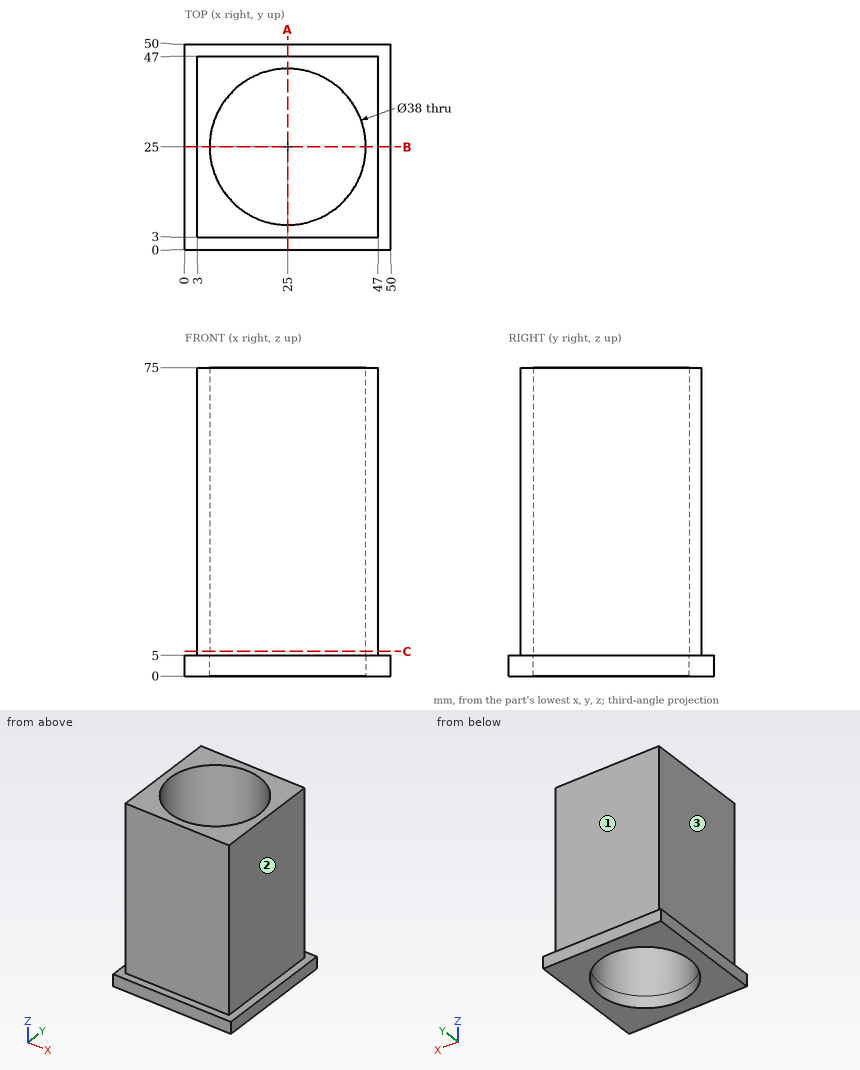
For this review, use the dimensioned drawing (mm, ordinates from the lowest corner) and the shaded views. A direction names the side the tool comes from. Coordinates: 2 decimals unless noted, no trailing zeros. Order: outer loops, then holes, each group sorted by start corner. A loop starts at its lowest first (then second) coordinate and runs counter-clockwise, first axis right, second up. Notation, with made-up numbers: M -19.5,-10 L 26.5,-10 A18 cw 26.5,6 Z; hole C 83.25,-22 d7. An arc over 180 degrees is marked long. Answer as a JSON object with one key per item and string values. Group by question number.
1) For pin 1 (6 mm diameter, centred on x = 24.5, z = 28.5, fed in from +Y); pin 2 (12 mm diameter, centred on x = 24.5, z = 29, fed in from -Y); pin 3 (12 mm diameter, centred on y = 15, z = 64.5, fed in from +X), all flat-tipped, find the tip position at first contact; note any pin that passes through.
2) Wall thickness on L1, parallel to Y at x = 25, z = 1; L2, parallel to Y at x = 25, z = 22.5; L3, parallel to Y at x = 45.5, z = 9: over which ranges is each line inside the solid? List them lowest first.
3) Tool access review of the marked faces 1, 2 and 3: name each direction out of +Z, -Z, +X, -X, +Y, -Y from which nothing blocks a thin tool from reaching the whole face with its end or side.
4) Add section A-A, the plane x = 25. Write out the cut boundary in (y, z).
5) Add section C-C, the plane z = 6. Write out the cut boundary in (x, y), then the cut area to 3 significant figures.
Computed values:
{
 "1": {"pin 1": "stops at y = 47", "pin 2": "stops at y = 3", "pin 3": "stops at x = 47"},
 "2": {"L1": "y = 0 to 6, 44 to 50", "L2": "y = 3 to 6, 44 to 47", "L3": "y = 3 to 47"},
 "3": {"face 1": "+Z, +X, -X, +Y", "face 2": "+Z, +X, +Y, -Y", "face 3": "+Z, -X, +Y, -Y"},
 "4": {"outline": "M 0,0 L 6,0 L 6,75 L 3,75 L 3,5 L 0,5 Z; M 44,0 L 50,0 L 50,5 L 47,5 L 47,75 L 44,75 Z"},
 "5": {"outline": "M 3,3 L 47,3 L 47,47 L 3,47 Z; hole C 25,25 d38", "area": "802 mm^2"}
}
